Autodesk Inventor part; units mm, degrees
ref_plane "YZ Plane" through (0, 0, 0) normal (1, 0, 0) x (0, 1, 0)
ref_plane "XZ Plane" through (0, 0, 0) normal (0, 1, 0) x (-1, 0, 0)
ref_plane "XY Plane" through (0, 0, 0) normal (0, 0, 1) x (1, 0, 0)
sketch "Sketch1" plane through (0, 0, 0) normal (0, 1, 0) x (-1, 0, 0)
  line L0 (0, 0) -> (-10, 0)
  line L1 (-10, 0) -> (-10, -150)
  line L2 (-10, -150) -> (0, -150)
  line L3 (0, -150) -> (0, 0)
  circle A0 centre (-5, -75) radius 3
  dimension "d0" = 10
  dimension "d1" = 150
  dimension "d2" = 6
  dimension "d5" = 75
extrude "Extrusion1" add sketch "Sketch1" along normal blind 5
sketch "Sketch2" plane through (0, 0, 0) normal (0, -1, 0) x (1, 0, 0)
  circle A0 centre (5, -75) radius 3
  point P0 (0, 0)
extrude "Extrusion2" add sketch "Sketch2" against normal blind 40
properties part number "enganche vertical rueda gusano"
CAD build for the part. Positions are in the model's coordinates, mm. A direction names the side the tool comes from. Coordinates: 2 decimals unless noted, no trailing zeros. Loops run counter-clockwise (first coordinate to the right, second up) from the corner with the lowest first, then second, coordinate; pieces in that order, holes last. Notation, with made-up numbers: (21, 61.25) -> (68, 61.25) arc R30 ccw to (68, 97.25) -> close; hole circle Ø10 at (4, 46). An arc over 180 degrees is marked (long way). One line per item, written item: value.
1. Slice it at A-A on x = 5. Write the cut outline in (y, z), and give its area (3 significant figures).
Answers:
outline: (0, -150) -> (5, -150) -> (5, -78) -> (40, -78) -> (40, -72) -> (5, -72) -> (5, 0) -> (0, 0) -> close
area: 960 mm^2
2. Slice it at D-D on z = -18. Write the cut outline in (x, y), and give its area (3 significant figures).
Answers:
outline: (0, 0) -> (10, 0) -> (10, 5) -> (0, 5) -> close
area: 50.0 mm^2
3. Which spindle directions (+Z, -Z, +X, -X, +Y, -Y) get a long thin tool onto all of the face, cutting with end or side? Do faces 1 (the face through (4.35, 22.26, -77.93)), 2 (the face through (10, 2, -74)). Say none if no direction does.
Answers:
face 1: +Y
face 2: +Z, -Z, +X, +Y, -Y
4. Flat gauge pins, fed straight in: P1, Ø3, axis at x = 8, y = 10, coming from the -Z side; P2, Ø5, axis at x = 7, y = 31, coming from the -Z side; P3, Ø4, axis at x = 3, y = 30, coming from the +Z side. Where does each tip first touch, or does it go through?
Answers:
P1: stops at z = -77.6
P2: stops at z = -78
P3: stops at z = -72
5. Slice it at B-B on z = -75. Write the cut outline in (x, y), and give its area (3 significant figures).
Answers:
outline: (0, 0) -> (10, 0) -> (10, 5) -> (8, 5) -> (8, 40) -> (2, 40) -> (2, 5) -> (0, 5) -> close
area: 260 mm^2
6. Slice it at C-C on y = 26. Write the cut outline in (x, z).
Answers:
outline: circle Ø6 at (5, -75)
7. Drill centre lines: line 1 (Y direction, x = 6.75, z = -18); line 2 (X direction, y = 21, z = -73); line 3 (Z direction, x = 5.5, y = 13). Where is each one in solid material? Low to high. Write a range as [from, to].
Answers:
line 1: y = [0, 5]
line 2: x = [2.76, 7.24]
line 3: z = [-77.96, -72.04]
